```python
from build123d import *

# Parameters (mm, degrees)
SKETCH1_W           = 50
SKETCH1_H           = 3
SKETCH1_W_2         = 3
SKETCH1_H_2         = 50
BOSS_EXTRUDE1_DEPTH = 3


with BuildPart() as part:
    # Sketch1 → Boss-Extrude1 (new body)
    with BuildSketch(Plane(origin=(0, 0, 0), x_dir=(1, 0, 0), z_dir=(0, 1, 0))):
        with BuildLine():
            Line((-55, 55), (55, 55))
            Line((55, 55), (55, -55))
            Line((55, -55), (42, -55))
            Line((42, -55), (42, -8))
            ThreePointArc((42, -8), (27.355339059, 27.355339059), (-8, 42))
            Line((-8, 42), (-55, 42))
            Line((-55, 42), (-55, 55))
        make_face()
        with Locations((-20, 48.5)):
            Rectangle(SKETCH1_W, SKETCH1_H, mode=Mode.SUBTRACT)
        with Locations((48.5, -20)):
            Rectangle(SKETCH1_W_2, SKETCH1_H_2, mode=Mode.SUBTRACT)
    extrude(amount=BOSS_EXTRUDE1_DEPTH)


solid = part.part
```
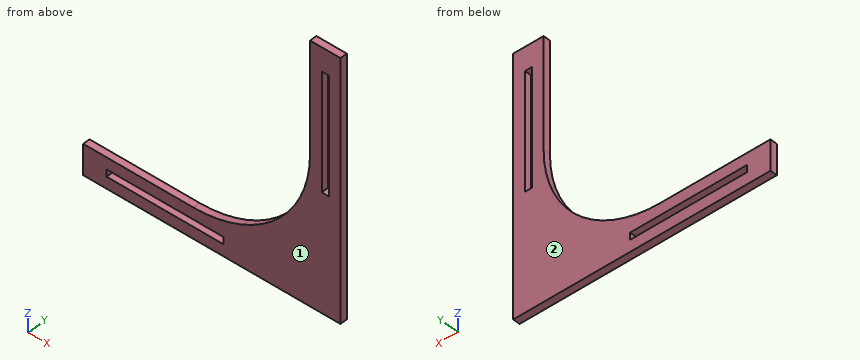
Work out the finished part from the listing and answer in its coordinate system (mm). Face numbers are marked on the shaded views. Round coordinates to 2 decimals unless told otherwise and drop trailing zeros. Write each loop counter-clockwise with the first axis right and the second up, starting at its lowest first coordinate (ties: lowest second). Pieces come first, ordered by that corner, then holes.
1) A cutting plane is placed at D-D on z = -36. Determine the outline of the cut face in (x, y), and give its area (3 significant figures).
2) A cutting plane is placed at A-A on z = 25.5. Determine the outline of the cut face in (x, y), and give its area (3 significant figures).
3) Determine the mould class of the marked faces 1 and 2 for opening direction Y: pulls with the +Y half, pulls with the -Y half, needs draft (parallel to the pull), parting line crosses it, or undercut.
4) Flat-ended cylindrical pins translate along their axes: P1, Ø0.9, axis at y = 1, z = 21, coming from the -X side; P2, Ø1.5, axis at x = 1, y = 2.5, coming from the +Z side; P3, Ø1.5, axis at x = -33, y = 1.5, coming from the +Z side. Find the tip coordinate at first contact, or state that the pin passes through.
5) Consider probe 1 along X at (y, z) = (2.7, -49.5); probe 2 along Z at (x, y) = (-40, 1.3); probe 3 along X at (y, z) = (0.65, 25). Determine where each line is inside the solid, lowest interval first.
6) A cutting plane is placed at B-B on x = -26.5. Determine the outline of the cut face in (y, z).
7) A cutting plane is placed at C-C on y = 2.1. Determine the outline of the cut face in (x, z).
Entries:
1. outline: (15.75, 0) - (55, 0) - (55, 3) - (15.75, 3) - close
1. area: 118 mm2
2. outline: (42, 0) - (47, 0) - (47, 3) - (42, 3) - close; (50, 0) - (55, 0) - (55, 3) - (50, 3) - close
2. area: 30.0 mm2
3. face 1: pulls with the -Y half
3. face 2: pulls with the +Y half
4. P1: stops at x = 42
4. P2: stops at z = -41.04
4. P3: stops at z = -42
5. probe 1: x = -55 to -45, 5 to 55
5. probe 2: z = -55 to -50, -47 to -42
5. probe 3: x = 42 to 47, 50 to 55
6. outline: (0, -55) - (3, -55) - (3, -50) - (0, -50) - close; (0, -47) - (3, -47) - (3, -42) - (0, -42) - close
7. outline: (-55, -55) - (55, -55) - (55, 55) - (42, 55) - (42, 8) arc R50 cw to (-8, -42) - (-55, -42) - close; hole (-45, -50) - (5, -50) - (5, -47) - (-45, -47) - close; hole (47, -5) - (50, -5) - (50, 45) - (47, 45) - close
